Can you work these out from the model? Positions are in its coordinate system, mm. A direction names the side the tool comes from. Round coordinates to 2 decimals unless told otherwise and drop trailing zeros. Loops run counter-clockwise (first coordinate to the right, second up) from the corner with the lowest first, then second, coordinate; pieces in that order, holes last. Notation, with made-up numbers: (89, 21) -> (134, 21) arc R24 cw to (134, 46) -> close; hole circle Ø4 at (87.5, 86.25). An arc over 180 degrees is marked (long way). Use a Markdown table: item, result.
from build123d import *

# Parameters (mm, degrees)
MAINBODY_EXTRUDE_START = -20
PROJECTIONXY_SKETCH_W  = 10.314570696
PROJECTIONXY_SKETCH_H  = 10.314570696
MAINBODY_EXTRUDE_DEPTH = 5
BORE_CUT_DEPTH         = 22.28838144
BORE_CUT_DEPTH_BACK    = 22.28838144
BORE_SKETCH_R          = 2.55
POSTS_EXTRUDE_START    = -20
POSTS_SKETCH_R         = 0.65
POSTS_EXTRUDE_DEPTH    = 40


with BuildPart() as part:
    # projectionXy_sketch → mainBody_extrude (new body)
    with BuildSketch(Plane.XY.offset(MAINBODY_EXTRUDE_START)):
        Rectangle(PROJECTIONXY_SKETCH_W, PROJECTIONXY_SKETCH_H)
    extrude(amount=MAINBODY_EXTRUDE_DEPTH)

    # bore_sketch → bore_cut (cut, two sides: drawn at the far end of the back side and taken through both)
    with BuildSketch(Plane.XY.offset(-BORE_CUT_DEPTH_BACK)):
        Circle(BORE_SKETCH_R)
    extrude(amount=BORE_CUT_DEPTH + BORE_CUT_DEPTH_BACK, mode=Mode.SUBTRACT)

    # posts_sketch → posts_extrude (add)
    with BuildSketch(Plane.XY.offset(POSTS_EXTRUDE_START)):
        with Locations((4.207285348, -4.207285348)):
            Circle(POSTS_SKETCH_R)
        with Locations((-4.207285348, -4.207285348)):
            Circle(POSTS_SKETCH_R)
        with Locations((-4.207285348, 4.207285348)):
            Circle(POSTS_SKETCH_R)
        with Locations((4.207285348, 4.207285348)):
            Circle(POSTS_SKETCH_R)
    extrude(amount=POSTS_EXTRUDE_DEPTH)


solid = part.part
1. I need wall thicknesses on line 1 (X direction, y = 0, z = -17.65); line 2 (Z direction, x = -4.25, y = -3.25). Which ranges of each line are inside material? Lowest first, please.
Answer sheet:
| item | result |
|---|---|
| line 1 | x = -5.16 to -2.55, 2.55 to 5.16 |
| line 2 | z = -20 to -15 |
2. I want a section at A-A (x = 0). Please give me the cut outline in (y, z).
Answer sheet:
| item | result |
|---|---|
| outline | (-5.16, -20) -> (-2.55, -20) -> (-2.55, -15) -> (-5.16, -15) -> close; (2.55, -20) -> (5.16, -20) -> (5.16, -15) -> (2.55, -15) -> close |
3. Which directions (+Z, -Z, +X, -X, +Y, -Y) give clear straight access to the entire face, cutting with the end or side of a thin tool? Please do faces 1 (the flat face through (0, 5.157, -18)), 2 (the cylindrical face through (4.81, 3.96, 2.25)).
Answer sheet:
| item | result |
|---|---|
| face 1 | +Z, -Z, +X, -X, +Y |
| face 2 | +Z |
4. I want a section at D-D (x = 3). Please give me the cut outline in (y, z).
Answer sheet:
| item | result |
|---|---|
| outline | (-5.16, -20) -> (5.16, -20) -> (5.16, -15) -> (-5.16, -15) -> close |
5. If we mould it in two halves opening along X, with no side actions, what happens to faces 3 (the flat face through (5.157, 0, -18)), 4 (the flat face through (-4, -4, 20)), 5 (the flat face through (-2, 2, -15))? For each: +X half, -X half, draft (parallel to the pull), parting line (faces both ways), or undercut.
Answer sheet:
| item | result |
|---|---|
| face 3 | +X half |
| face 4 | draft |
| face 5 | undercut |
6. I want a section at C-C (z = -17). Please give me the cut outline in (x, y).
Answer sheet:
| item | result |
|---|---|
| outline | (-5.16, -5.16) -> (5.16, -5.16) -> (5.16, 5.16) -> (-5.16, 5.16) -> close; hole circle Ø5.1 at (0, 0) |
7. Will these pins go through, and if not, where does the flat tip stop? pin 1 Ø3 at (x, y) = (-0.5, -1) entering from +Z; pin 2 Ø1.5 at (y, z) = (3, -1.5) entering from -X.
Answer sheet:
| item | result |
|---|---|
| pin 1 | stops at z = -15 |
| pin 2 | stops at x = -4.67 |
